```python
from build123d import *

# Parameters (mm, degrees)
EXTRUDE_1_DEPTH     = 5
SKETCH_3_R          = 12.5
EXTRUDE_2_DEPTH     = 11
CHAMFER_1_SIZE      = 1.5
EXTRUDE_START       = 3
SKETCH_4_R          = 12.5
EXTRUDE_3_DEPTH     = 3
EXTRUDE_4_DEPTH     = 14
SKETCH_6_R          = 12.458994032
EXTRUDE_5_DEPTH     = 6
FILLET_1_R          = 6
SKETCH_7_R          = 6.574183754
CUT_EXTRUDE_1_DEPTH = 42
FILLET_2_R          = 2


with BuildPart() as part:
    # Эскиз2 → Бобышка-Вытянуть1 (new body)
    with BuildSketch(Plane.XY):
        Polygon((12.704765165, -7.974267497), (13.258300811, 7.015515633), (0.553535647, 14.98978313), (-12.704765165, 7.974267497), (-13.258300811, -7.015515633), (-0.553535647, -14.98978313), align=None)
    extrude(amount=EXTRUDE_1_DEPTH)

    # Эскиз3 → Бобышка-Вытянуть2 (add)
    with BuildSketch(Plane(origin=(0, 0, 0), x_dir=(-1, 0, 0), z_dir=(0, 0, -1))):
        with Locations(Location((0, 0, 0), (0, 0, 180))):
            Circle(SKETCH_3_R)
    extrude(amount=EXTRUDE_2_DEPTH)

    # Фаска1
    chamfer_1_edges = [part.edges().sort_by_distance(p)[0] for p in [
        (-12.5, 0, -11),
    ]]
    chamfer(chamfer_1_edges, length=CHAMFER_1_SIZE)

    # Эскиз4 → Бобышка-Вытянуть3 (add)
    with BuildSketch(Plane.XY.offset(5).offset(EXTRUDE_START)):
        Circle(SKETCH_4_R)
    extrude(amount=-EXTRUDE_3_DEPTH)

    # Эскиз5 → Бобышка-Вытянуть4 (add)
    with BuildSketch(Plane.XY.offset(8)):
        Polygon((12.559385181, 7.335539252), (-0.073070753, 14.544516248), (-12.632455933, 7.208976996), (-12.559385181, -7.335539252), (0.073070753, -14.544516248), (12.632455933, -7.208976996), align=None)
    extrude(amount=EXTRUDE_4_DEPTH)

    # Эскиз6 → Бобышка-Вытянуть5 (add)
    with BuildSketch(Plane.XY.offset(22)):
        Circle(SKETCH_6_R)
    extrude(amount=EXTRUDE_5_DEPTH)

    # Скругление1
    fillet_1_edges = [part.edges().sort_by_distance(p)[0] for p in [
        (-12.458994032, 0, 28),
    ]]
    fillet(fillet_1_edges, radius=FILLET_1_R - 0.0001)  # a hair under: the kernel refuses the full size

    # Эскиз7 → Вырез-Вытянуть1 (cut)
    with BuildSketch(Plane.XY.offset(28)):
        with Locations(Location((0, 0, 0), (0, 0, 180))):
            Circle(SKETCH_7_R)
    extrude(amount=-CUT_EXTRUDE_1_DEPTH, mode=Mode.SUBTRACT)

    # Скругление2
    fillet_2_edges = [part.edges().sort_by_distance(p)[0] for p in [
        (-0.553535647, -14.98978313, 2.5),
        (-13.258300811, -7.015515633, 2.5),
        (-12.704765165, 7.974267497, 2.5),
        (0.553535647, 14.98978313, 2.5),
        (13.258300811, 7.015515633, 2.5),
        (12.704765165, -7.974267497, 2.5),
        (12.632455933, -7.208976996, 15),
        (12.559385181, 7.335539252, 15),
        (-0.073070753, 14.544516248, 15),
        (-12.632455933, 7.208976996, 15),
        (-12.559385181, -7.335539252, 15),
        (0.073070753, -14.544516248, 15),
    ]]
    fillet(fillet_2_edges, radius=FILLET_2_R)


solid = part.part
```
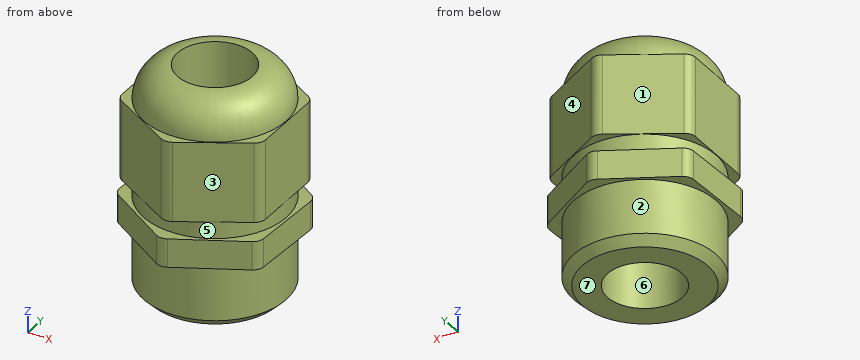
Build history of the part. All positions in model axes, mm. Face numbers are marked on the shaded views. A direction names the side the tool comes from. Give positions to 0.01 mm unless a question says otherwise; leave off trailing zeros. Order: outer loops, then holes, each group sorted by start corner. A loop starts at its lowest first (then second) coordinate and runs counter-clockwise, first axis right, second up. Notation, with made-up numbers: M -20.5,56.25 L -0.5,56.25 A18 cw -0.5,61.25 Z; hole C 38.25,30.5 d2. An arc over 180 degrees is marked long. Return JSON: item names as keys, results as strings.
Q1. Flat gauge pins, fed straight in: pin 1 (5 mm diameter, centred on y = 0.5, z = 6.5, fed in from -X); pin 2 (4 mm diameter, centred on y = -5.5, z = 15, fed in from +X); pin 3 (8 mm diameter, centred on y = 11, z = 15.5, fed in from +X). Where does each tip first touch, or does it go through?
Answer list:
{"pin 1": "stops at x = -13.05", "pin 2": "stops at x = 12.63", "pin 3": "stops at x = 12.39"}
Q2. Two-plate mould, pull along X, no slides. Class the marked faces 5, 6 and 7: pulls with the +X half, pulls with the -X half, needs draft (parallel to the pull), parting line crosses it, or undercut.
Answer list:
{"face 5": "parting line crosses it", "face 6": "undercut", "face 7": "needs draft"}
Q3. Wall check: probe 1 along Z at (x, y) = (11.5, 5.25); probe 2 along Y at (x, z) = (0, 7.5); probe 3 along Y at (x, z) = (0, 15.5). Give the ranges that are in metal, low to high. Write a range as from..to.
Answer list:
{"probe 1": "z = 0..5, 8..22", "probe 2": "y = -12.5..-6.57, 6.57..12.5", "probe 3": "y = -14.23..-6.57, 6.57..14.23"}
Q4. Band-saw the part on D-D (z = -3.5). Give the cut face in (x, y).
Answer list:
{"outline": "C 0,0 d25; hole C 0,0 d13.15"}
Q5. 3-axis set-ups, long thin cutter, end or side, ignore diameter. For the marked faces 1, 2, 3 and 4: which of +Z, -Z, +X, -X, +Y, -Y reach the whole face in a straight line?
Answer list:
{"face 1": "+Z, -X, +Y", "face 2": "-Z", "face 3": "+Z, +X, -Y", "face 4": "+Z, +X, +Y"}
Q6. Band-saw the part on A-A (z = 3). Give the cut face in (x, y), then the cut area to 3 significant figures.
Answer list:
{"outline": "M -13.22,-5.86 A2 ccw -12.28,-7.63 L -1.53,-14.38 A2 ccw 0.47,-14.45 L 11.68,-8.51 A2 ccw 12.75,-6.82 L 13.22,5.86 A2 ccw 12.28,7.63 L 1.53,14.38 A2 ccw -0.47,14.45 L -11.68,8.51 A2 ccw -12.75,6.82 Z; hole C 0,0 d13.15", "area": "447 mm^2"}
